Design review of the part built by this model. Coordinates are the model's own, in mm. A direction names the side the tool comes from. Round coordinates to 2 decimals unless told otherwise and drop trailing zeros. Loops run counter-clockwise (first coordinate to the right, second up) from the corner with the lowest first, then second, coordinate; pieces in that order, holes last. Notation, with made-up numbers: (77.25, 26.5) - (127.25, 26.5) arc R24 ccw to (127.25, 55.5) - close; hole circle Ø9 at (34, 60.25). An arc over 180 degrees is marked (long way). Use one line per item in the form item = value. Start each with the question number.
(1) We need section D-D, the plane x = 19. Write out the cut boundary in (y, z) (3 decimals), then the cut area to 3 significant figures.
(2) The part is to be moulded in two halves that separate along Y. For faces 1 (the flat face through (13, 12.7, 2)), 2 (the flat face through (2, -6.35, 2)), 3 (the cylindrical face through (24.74, -6.15, 1.61)), say which applies: released by +Y, released by -Y, zero draft, split by the parting line, or undercut.
(3) We need section B-B, the plane z = 2.65. Write out the cut boundary in (x, y) (3 decimals).
(4) Wall thickness on probe 1 along X at (y, z) = (-10, 0.9) (3 decimals); probe 2 along Y at (x, z) = (21, 2.45); probe 3 along X at (y, z) = (-7.25, 1.75) (1 decimal): over which ranges is each line inside the solid? List them lowest first. Write a range as [from, to].
(5) We need section C-C, the plane x = 4. Write out the cut boundary in (y, z) (3 decimals), then the cut area to 3 significant figures.
(6) We need section A-A, the plane x = 24. Write out the cut boundary in (y, z) (3 decimals).
(7) Machinability: for faces 4 (the flat face through (16, -1, 0)), 5 (the flat face through (2, 6.35, 2)), 6 (the flat face through (3.175, -10, 2)), which of the approach directions +Z, -Z, +X, -X, +Y, -Y give a long, thin tool a straight path to every point of the face, cutting with its end or side? Answer none if there is none.
(8) For pin 1 (1.6 mm diameter, centred on x = 2, z = 2, fed in from +Y); pin 2 (1.6 mm diameter, centred on y = 10, z = 2, fed in from -X) (3 decimals), all flat-tipped, find the tip position at first contact; note any pin that passes through.
from build123d import *

# Parameters (mm, degrees)
BOSS_EXTRUDE1_DEPTH = 3.175
SKETCH2_R           = 3.302
CUT_EXTRUDE1_DEPTH  = 3.175
FILLET1_R           = 9.525
SKETCH3_W           = 3.175
SKETCH3_H           = 6.35
CUT_EXTRUDE2_DEPTH  = 3.175


with BuildPart() as part:
    # Sketch1 → Boss-Extrude1 (new body)
    with BuildSketch(Plane.XY):
        Polygon((0, 12.7), (0, -12.7), (9.525, -12.7), (31.75, -15.875), (31.75, 12.7), align=None)
    extrude(amount=BOSS_EXTRUDE1_DEPTH)

    # Sketch2 → Cut-Extrude1 (cut)
    with BuildSketch(Plane.XY.offset(3.175)):
        with Locations((21.588299978, -7.140871599)):
            Circle(SKETCH2_R)
    extrude(amount=-CUT_EXTRUDE1_DEPTH, mode=Mode.SUBTRACT)

    # Fillet1
    fillet1_edges = [part.edges().sort_by_distance(p)[0] for p in [
        (31.75, 12.7, 1.5875),
        (31.75, -15.875, 1.5875),
        (9.525, -12.7, 1.5875),
    ]]
    fillet(fillet1_edges, radius=FILLET1_R)

    # Sketch3 → Cut-Extrude2 (cut)
    with BuildSketch(Plane.XY.offset(3.175)):
        with Locations((1.5875, -9.525)):
            Rectangle(SKETCH3_W, SKETCH3_H)
        with Locations((1.5875, 9.525)):
            Rectangle(SKETCH3_W, SKETCH3_H)
    extrude(amount=-CUT_EXTRUDE2_DEPTH, mode=Mode.SUBTRACT)


solid = part.part
Data:
q1.outline = (-14.054, 0) - (-9.191, 0) - (-9.191, 3.175) - (-14.054, 3.175) - close; (-5.091, 0) - (12.7, 0) - (12.7, 3.175) - (-5.091, 3.175) - close
q1.area = 71.9 mm^2
q2.face_1 = released by +Y
q2.face_2 = released by -Y
q2.face_3 = undercut
q3.outline = (0, -6.35) - (3.175, -6.35) - (3.175, -12.7) - (8.848, -12.7) arc R9.525 cw to (10.195, -12.796) - (20.878, -14.322) arc R9.525 ccw to (31.75, -4.893) - (31.75, 3.175) arc R9.525 ccw to (22.225, 12.7) - (3.175, 12.7) - (3.175, 6.35) - (0, 6.35) - close; hole circle Ø6.604 at (21.588, -7.141)
q4.probe_1 = [3.175, 19.936], [23.24, 30.265]
q4.probe_2 = [-14.34, -10.39], [-3.89, 12.7]
q4.probe_3 = [3.2, 18.3], [24.9, 31.5]
q5.outline = (-12.7, 0) - (12.7, 0) - (12.7, 3.175) - (-12.7, 3.175) - close
q5.area = 80.6 mm^2
q6.outline = (-14.251, 0) - (-9.396, 0) - (-9.396, 3.175) - (-14.251, 3.175) - close; (-4.885, 0) - (12.533, 0) - (12.533, 3.175) - (-4.885, 3.175) - close
q7.face_4 = -Z, +X, -X, +Y, -Y
q7.face_5 = +Z, -Z, -X, +Y
q7.face_6 = +Z, -Z, -X, -Y
q8.pin_1 = 6.35
q8.pin_2 = 3.175
